Could you check a few things on this model? Use its own coordinates, in mm. A direction names the side the tool comes from. Coordinates: 2 decimals unless noted, no trailing zeros. Loops run counter-clockwise (first coordinate to the right, second up) from the corner with the lowest first, then second, coordinate; pieces in that order, holes last. Notation, with made-up numbers: (23, 86) - (78, 86) arc R31 ccw to (78, 119) - close; hole circle Ø2 at (-2, 8.25). An arc over 180 degrees is marked (long way). Use CSV: the item, a comma, the result in double quotes.
from build123d import *

# Parameters (mm, degrees)
SKETCH1_R           = 1.85
BOSS_EXTRUDE1_DEPTH = 1.524
SKETCH2_W           = 10.16
SKETCH2_H           = 9
BOSS_EXTRUDE2_DEPTH = 3.5
SKETCH3_R           = 0.75
BOSS_EXTRUDE3_DEPTH = 4
SKETCH6_R           = 0.46355
BOSS_EXTRUDE6_DEPTH = 2


with BuildPart() as part:
    # Sketch1 → Boss-Extrude1 (new body)
    with BuildSketch(Plane.XZ.offset(-165.590407598)):
        Polygon((-4.08, 15.5), (-5.08, 13.5), (-5.08, 0), (5.08, 0), (5.08, 13.5), (4.08, 15.5), align=None)
        with Locations(Location((0, 12.5, 0), (0, 0, 90))):
            Circle(SKETCH1_R, mode=Mode.SUBTRACT)
    extrude(amount=-BOSS_EXTRUDE1_DEPTH)

    # Sketch2 → Boss-Extrude2 (add)
    with BuildSketch(Plane.XZ.offset(-165.590407598)):
        with Locations((0, 4.5)):
            Rectangle(SKETCH2_W, SKETCH2_H)
    extrude(amount=BOSS_EXTRUDE2_DEPTH)

    # Sketch3 → Boss-Extrude3 (add)
    with BuildSketch(Plane(origin=(0, 0, 0), x_dir=(-1, 0, 0), z_dir=(0, 0, -1))):
        with Locations(Location((2.54, 164.090407598, 0), (0, 0, 180))):
            Circle(SKETCH3_R)
        with Locations((0, 164.090407598)):
            Circle(SKETCH3_R)
        with Locations((-2.54, 164.090407598)):
            Circle(SKETCH3_R)
    extrude(amount=BOSS_EXTRUDE3_DEPTH)

    # Sketch6 → Boss-Extrude6 (add)
    with BuildSketch(Plane(origin=(0, 0, -4), x_dir=(-1, 0, 0), z_dir=(0, 0, -1))):
        with Locations(Location((2.54, 164.090407598, 0), (0, 0, 180))):
            Circle(SKETCH6_R)
        with Locations((0, 164.090407598)):
            Circle(SKETCH6_R)
        with Locations((-2.54, 164.090407598)):
            Circle(SKETCH6_R)
    extrude(amount=BOSS_EXTRUDE6_DEPTH)


solid = part.part
(1) Which directions (+Z, -Z, +X, -X, +Y, -Y) give clear straight access to the entire face, cutting with the end or side of a thin tool? Please do faces 5 (the face through (-1.2, 165.59, 10.9)), 6 (the face through (0.71, 166.34, 14.21)), 7 (the face through (0.06, 164.55, -4.99)).
Computed:
face 5,"+Z, +X, -X, -Y"
face 6,"+Y, -Y"
face 7,"-Z"
(2) Suppose I cut it at A-A (z = 12.5). Write out the boundary of the cut face in (x, y), plus the area to 3 significant figures.
Computed:
outline,"(-5.08, 165.59) - (-1.85, 165.59) - (-1.85, 167.11) - (-5.08, 167.11) - close; (1.85, 165.59) - (5.08, 165.59) - (5.08, 167.11) - (1.85, 167.11) - close"
area,"9.85 mm²"
(3) Thinking about a two-plate mould opening in X: for faces 1 (the face through (2.638, 164.834, -1.972)), 2 (the face through (-5.08, 165, 5)), 3 (the face through (-2.638, 163.347, -1.972)), 4 (the face through (0, 164, 9)), which applies, +X half, -X half, draft (parallel to the pull), parting line (faces both ways), or undercut?
Computed:
face 1,"undercut"
face 2,"-X half"
face 3,"undercut"
face 4,"draft"
(4) Please list where these lines run through material, in increasing order: line 1 (X direction, y = 166.4, z = 12.5); line 2 (Z direction, x = 1, y = 163.5); line 3 (Y direction, x = -2, z = 11.5).
Computed:
line 1,"x = -5.08 to -1.85, 1.85 to 5.08"
line 2,"z = 0 to 9"
line 3,"y = 165.59 to 167.11"
(5) Suppose I cut it at B-B (y = 166.1). Write out the boundary of the cut face in (x, z), plus the area to 3 significant figures.
Computed:
outline,"(-5.08, 0) - (5.08, 0) - (5.08, 13.5) - (4.08, 15.5) - (-4.08, 15.5) - (-5.08, 13.5) - close; hole circle Ø3.7 at (0, 12.5)"
area,"145 mm²"
(6) Suppose I cut it at D-D (x = 2.54). Write out the boundary of the cut face in (y, z), plus the area to 3 significant figures.
Computed:
outline,"(162.09, 0) - (163.34, 0) - (163.34, -4) - (163.63, -4) - (163.63, -6) - (164.55, -6) - (164.55, -4) - (164.84, -4) - (164.84, 0) - (167.11, 0) - (167.11, 15.5) - (165.59, 15.5) - (165.59, 9) - (162.09, 9) - close"
area,"63.0 mm²"
(7) Suppose I cut it at C-C (x = 1). Write out the boundary of the cut face in (y, z).
Computed:
outline,"(162.09, 0) - (167.11, 0) - (167.11, 10.94) - (165.59, 10.94) - (165.59, 9) - (162.09, 9) - close; (165.59, 14.06) - (167.11, 14.06) - (167.11, 15.5) - (165.59, 15.5) - close"
(8) Will these pins go through, and if not, where does the flat tip stop? pin 1 (1.2 mm diameter, centred on x = 0.5, y = 164, fed in from -Z); pin 2 (1.5 mm diameter, centred on y = 163, z = -1, fed in from +X); pin 3 (2 mm diameter, centred on x = 1, z = 12.5, fed in from -Y).
Computed:
pin 1,"stops at z = -6"
pin 2,"stops at x = 3.21"
pin 3,"stops at y = 165.59"
